Geometry check sheet. Reference: drawing and pictorial views, mm from the part's lowest x, y, z. A direction names the side the tool comes from. Give positions to 0.01 mm unless a question says otherwise; leave off trailing zeros. Order: outer loops, then holes, each group sorted by start corner. A loop starts at its lowest first (then second) coordinate and runs counter-clockwise, first axis right, second up. Notation, with made-up numbers: (87, -6) -> (141, -6) arc R12 cw to (141, 7) -> close; hole circle Ø8 at (51.5, 22). An arc over 180 degrees is marked (long way). Write each question's results on one line, items separated by ' | '. Start each with the question number.
1. Set-up check for the marked faces 1, 2 and 3: record each of +Z, -Z, +X, -X, +Y, -Y from which the full face is reachable in a straight line by a thin tool's end or side.
2. Depth check by flat-ended pin: pin 1 Ø7.5 at (y, z) = (10.5, 10.5) entering from +X; pin 2 Ø10.5 at (x, z) = (10, 12.5) entering from -Y; pin 3 Ø4 at (x, y) = (15.5, 11) entering from +Z. Enter the tip coordinate at first touch or a pass-through.
3. Material ranges on L1, parallel to Z at x = 42, y = 16.6 (3 decimals); L2, parallel to Y at x = 4.75, z = 2.85 (3 decimals); L3, parallel to Z at x = 22.5, y = 5, recorded low to high. Write a range as from..to.
4. Cross-section at A-A, the plane y = 11.9. Enter the section's corners in (x, z) (3 decimals).
5. Cross-section at B-B, the plane x = 42. Enter the section's corners in (y, z) (3 decimals), then the cut area to 3 significant figures.
6. Cross-section at C-C, the plane x = 4.75. Enter the section's corners in (y, z) (3 decimals).
7. Cross-section at D-D, the plane x = 33. Enter the section's corners in (y, z) (3 decimals), then the cut area to 3 significant figures.
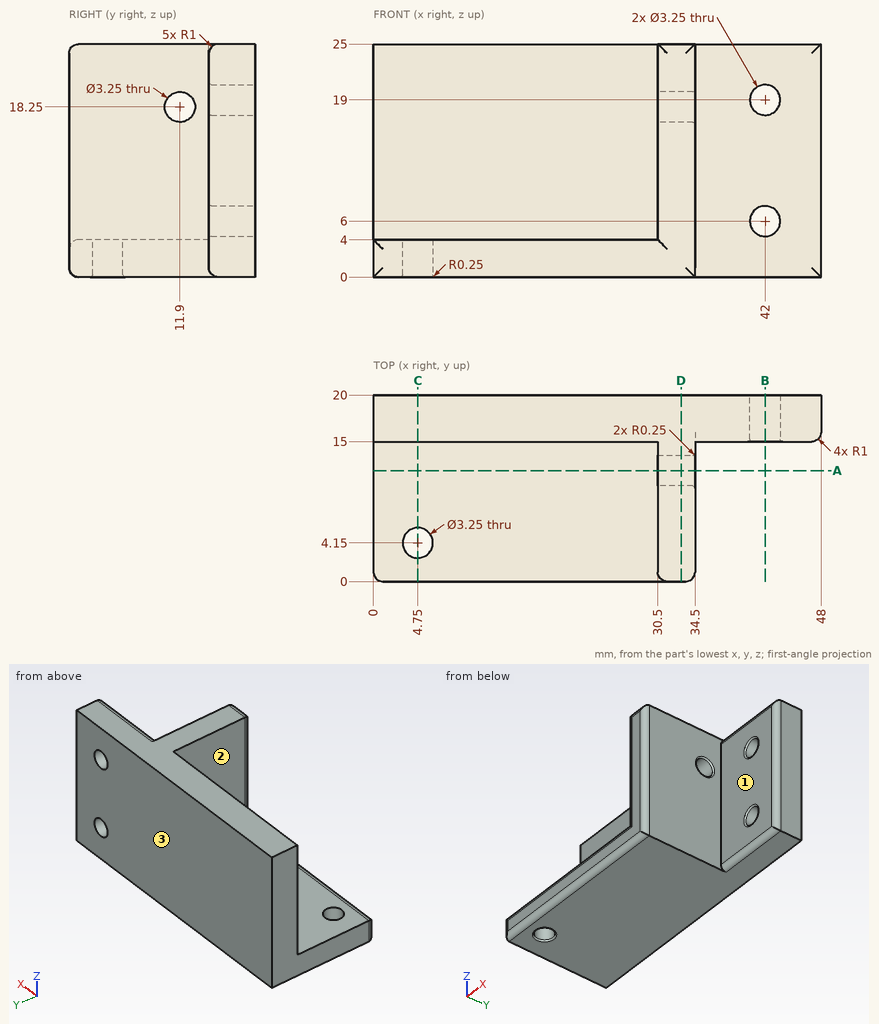
Results below:
1) face 1: +Z, -Z, +X, -Y | face 2: +Z, -X, -Y | face 3: +Z, -Z, +X, -X, +Y
2) pin 1: stops at x = 34.5 | pin 2: stops at y = 15 | pin 3: stops at z = 4
3) L1: z = 0..4.375, 7.625..17.375, 20.625..25 | L2: y = 0..2.525, 5.775..20 | L3: z = 0..4
4) outline: (0, 0) -> (34.5, 0) -> (34.5, 16.375) arc R0.25 ccw to (34.25, 16.625) -> (30.5, 16.625) -> (30.5, 4) -> (0, 4) -> close; (30.5, 19.875) -> (34.25, 19.875) arc R0.25 ccw to (34.5, 20.125) -> (34.5, 25) -> (30.5, 25) -> close
5) outline: (15, 1) arc R1 ccw to (16, 0) -> (20, 0) -> (20, 4.375) -> (15.25, 4.375) arc R0.25 ccw to (15, 4.125) -> close; (15, 7.875) arc R0.25 ccw to (15.25, 7.625) -> (20, 7.625) -> (20, 17.375) -> (15.25, 17.375) arc R0.25 ccw to (15, 17.125) -> close; (15, 20.875) arc R0.25 ccw to (15.25, 20.625) -> (20, 20.625) -> (20, 25) -> (16, 25) arc R1 ccw to (15, 24) -> close | area: 92.0 mm²
6) outline: (0, 1) arc R1 ccw to (1, 0) -> (2.275, 0) arc R0.25 ccw to (2.525, 0.25) -> (2.525, 4) -> (1, 4) arc R1 ccw to (0, 3) -> close; (5.775, 0.25) arc R0.25 ccw to (6.025, 0) -> (20, 0) -> (20, 25) -> (15, 25) -> (15, 4) -> (5.775, 4) -> close
7) outline: (0, 1) arc R1 ccw to (1, 0) -> (20, 0) -> (20, 25) -> (1, 25) arc R1 ccw to (0, 24) -> close; hole circle Ø3.25 at (11.9, 18.25) | area: 491 mm²
